Build history of the part. All positions in model axes, mm. Face numbers are marked on the shaded views. Give positions to 0.01 mm unless a question says otherwise; leave off trailing zeros. Write each loop counter-clockwise with the first axis right and the second up, starting at its lowest first coordinate (ties: lowest second). Pieces come first, ordered by that corner, then holes. Notation, with made-up numbers: M 68.5,33 L 109.5,33 A22 ccw 109.5,54 Z; hole C 39,35.25 d2. An arc over 180 degrees is marked long. One line per item, written item: value. Start each with the question number.
from build123d import *

# Parameters (mm, degrees)
SKETCH2_R           = 7.5
BOSS_EXTRUDE1_DEPTH = 13.5
SKETCH3_R           = 5
CUT_EXTRUDE1_DEPTH  = 5
FILLET1_R           = 7.5
THREAD1_PITCH       = 2
SKETCH10_W          = 14.918293933
SKETCH10_H          = 11.930208352
CUT_EXTRUDE2_DEPTH  = 5


with BuildPart() as part:
    # Sketch2 → Boss-Extrude1 (new body)
    with BuildSketch(Plane(origin=(0, 0, 0), x_dir=(1, 0, 0), z_dir=(0, 1, 0))):
        with Locations(Location((0, 0, 0), (0, 0, 270))):
            Circle(SKETCH2_R)
    extrude(amount=BOSS_EXTRUDE1_DEPTH)

    # Sketch3 → Cut-Extrude1 (cut)
    with BuildSketch(Plane(origin=(0, 0, 0), x_dir=(-1, 0, 0), z_dir=(0, -1, 0))):
        with Locations(Location((0, 0, 0), (0, 0, 90))):
            Circle(SKETCH3_R)
    extrude(amount=-CUT_EXTRUDE1_DEPTH, mode=Mode.SUBTRACT)

    # Fillet1
    fillet1_edges = [part.edges().sort_by_distance(p)[0] for p in [
        (0, 13.5, -7.5),
    ]]
    fillet(fillet1_edges, radius=FILLET1_R)

    # Thread1: the profile of Thread Profile2 profile screwed along a right-hand helix of 2.5 turns, 10 arcs to a turn; built about Z, then put on its axis
    thread1_z = Axis((0, 0, 0), (0, 0, 1))
    thread1_corners = [(5.0003, -1e-09, -0.000173205), (5.0003, -1e-09, 1.7501732), (3.91746825, -1e-09, 1.124999997), (3.91746825, -1e-09, 0.624999997)]
    with BuildLine(mode=Mode.PRIVATE) as thread1_profile:
        Line(thread1_corners[0], thread1_corners[1])
        Line(thread1_corners[1], thread1_corners[2])
        Line(thread1_corners[2], thread1_corners[3])
        Line(thread1_corners[3], thread1_corners[0])
    thread1_cap = Face(thread1_profile.wire())
    thread1_turn_angles = [0, 18, 36, 54, 72, 90, 108, 126, 144, 162, 180, 198, 216, 234, 252, 270, 288, 306, 324, 342, 360]
    thread1_turn_weights = [1, 0.9510565162951535, 1, 0.9510565162951535, 1, 0.9510565162951535, 1, 0.9510565162951535, 1, 0.9510565162951535, 1, 0.9510565162951535, 1, 0.9510565162951535, 1, 0.9510565162951535, 1, 0.9510565162951535, 1, 0.9510565162951535, 1]
    thread1_turn_rails = [Edge.make_bspline([Vector(p[0], p[1], 0).rotate(thread1_z, thread1_turn_angles[k]) / thread1_turn_weights[k] + Vector(0, 0, p[2] + THREAD1_PITCH * thread1_turn_angles[k] / 360) for k in range(21)], [0, 0, 0, 1, 1, 2, 2, 3, 3, 4, 4, 5, 5, 6, 6, 7, 7, 8, 8, 9, 9, 10, 10, 10], 2, thread1_turn_weights) for p in thread1_corners]
    thread1_turn_sides = [Face.make_surface_from_curves(thread1_turn_rails[p[0]], thread1_turn_rails[p[1]]) for p in [(0, 1), (1, 2), (2, 3), (3, 0)]]
    thread1_last_angles = [720, 738, 756, 774, 792, 810, 828, 846, 864, 882, 900]
    thread1_last_weights = [1, 0.9510565162951535, 1, 0.9510565162951535, 1, 0.9510565162951535, 1, 0.9510565162951535, 1, 0.9510565162951539, 1]
    thread1_last_rails = [Edge.make_bspline([Vector(p[0], p[1], 0).rotate(thread1_z, thread1_last_angles[k]) / thread1_last_weights[k] + Vector(0, 0, p[2] + THREAD1_PITCH * thread1_last_angles[k] / 360) for k in range(11)], [0, 0, 0, 1, 1, 2, 2, 3, 3, 4, 4, 5, 5, 5], 2, thread1_last_weights) for p in thread1_corners]
    thread1_last_sides = [Face.make_surface_from_curves(thread1_last_rails[p[0]], thread1_last_rails[p[1]]) for p in [(0, 1), (1, 2), (2, 3), (3, 0)]]
    thread1 = Plane(origin=(0, -1, 0), x_dir=(0.996194698, 0, -0.087155743), z_dir=(0, 1, 0)) * Solid(Shell([*[p.moved(Location((0, 0, THREAD1_PITCH * i))) for i in range(2) for p in thread1_turn_sides], *thread1_last_sides, thread1_cap, thread1_cap.rotate(thread1_z, 900).moved(Location((0, 0, THREAD1_PITCH * 900 / 360)))]))
    add(thread1)

    # Sketch10 → Cut-Extrude2 (cut)
    with BuildSketch(Plane(origin=(0, 0, 0), x_dir=(-1, 0, 0), z_dir=(0, -1, 0))):
        with Locations((1.239502166, -0.263539638)):
            Rectangle(SKETCH10_W, SKETCH10_H)
    extrude(amount=CUT_EXTRUDE2_DEPTH, mode=Mode.SUBTRACT)


solid = part.part
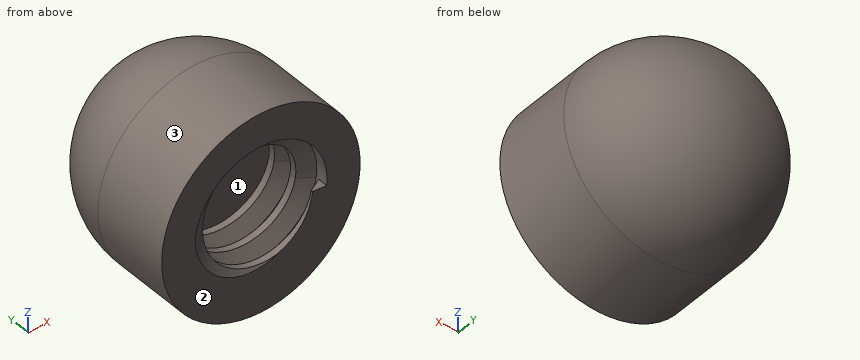
1) Band-saw the part on A-A (x = 6). List the corners of the cut face in (y, z), then the cut area to 3 significant figures.
2) Probe line 1 along X through (y, z) = (0.65, 0); line 2 along Z through (x, y) = (0, 2.7). List the from-to ranges inside material, lowest first. Write a range as from..to.
3) Band-saw the part on C-C (y = 8.75). List the corners of the cut face in (x, z), then the cut area to 3 significant figures.
4) Drop flat-ended pins along their axis: P1, Ø8, axis at x = 2.5, z = 5.5, coming from the -Y side; P2, Ø5, axis at x = -5.5, z = 4, coming from the +Y side; P3, Ø2, axis at x = 2.5, z = 5, coming from the +Y side; P4, Ø4, axis at x = 1.5, z = 1, coming from the -Y side. Give the stop position or say it passes through.
5) Band-saw the part on B-B (z = 6). List the corners of the cut face in (x, y).
6) Band-saw the part on D-D (y = 6.25). List the corners of the cut face in (x, z), then the cut area to 3 significant figures.
7) Mould opens along Y. For the marked faces 1, 2 and 3 say: released by +Y, released by -Y, zero draft, split by the parting line, or undercut.
Model answer:
1. outline: M 0,-4.5 L 6,-4.5 A4.5 ccw 6,4.5 L 0,4.5 Z
1. area: 85.8 mm²
2. line 1: x = -7.5..-3.92, 5..7.5
2. line 2: z = -7.5..-4.1, 4.6..7.5
3. outline: C 0,0 d13.96
3. area: 153 mm²
4. P1: stops at y = 0
4. P2: stops at y = 12.14
4. P3: stops at y = 11.93
4. P4: stops at y = 5
5. outline: M -4.5,0 L 4.5,0 L 4.5,6 A4.5 ccw -4.5,6 Z
6. outline: C 0,0 d14.99
6. area: 177 mm²
7. face 1: undercut
7. face 2: released by -Y
7. face 3: zero draft
